Build history of the part. All positions in model axes, mm. Face numbers are marked on the shaded views. Coordinates: 2 decimals unless noted, no trailing zeros. Order: outer loops, then holes, each group sorted by start corner. A loop starts at its lowest first (then second) coordinate and runs counter-clockwise, first axis right, second up. Notation, with made-up numbers: (72.25, 44.5) - (93.25, 44.5) arc R25 ccw to (93.25, 74.5) - close; hole circle Ø8 at (-13.5, 46). An arc over 180 degrees is marked (long way). Return JSON: item names as keys, results as strings.
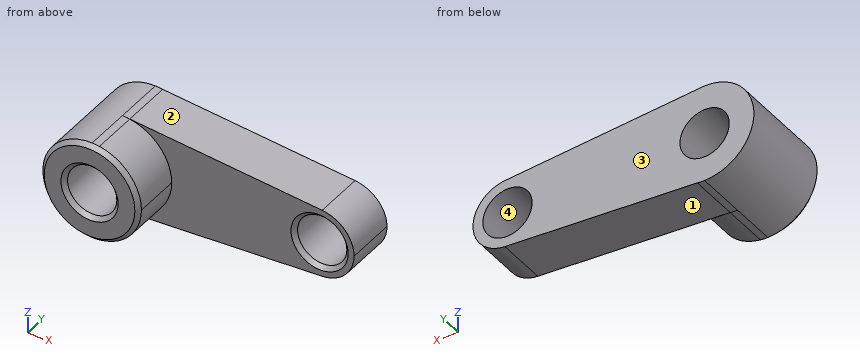
from build123d import *

# Parameters (mm, degrees)
F0_R        = 12.5
F1_DEPTH    = 25
F2_DEPTH    = 50
F3_T4_ANGLE = 203.6133668192
F3_T6_ANGLE = 179.9906971182


# Not quite as in the source:
# - a fillet or chamfer that OpenCascade refuses, or shapes differently, is made with other operations: its cross-section is extruded or revolved along the edge and cut away or added


with BuildPart() as f1:
    # F0 (on Front) → F1 (new body)
    with BuildSketch(Plane.XZ):
        with BuildLine():
            Line((3.7051688109, 24.7239099675), (0, 25))
            ThreePointArc((0, 25), (-25, 0), (0, -25))
            Line((0, -25), (3.7051688109, -24.7239099675))
            ThreePointArc((3.7051688109, -24.7239099675), (18.9424024383, -16.3151889313), (25, 0))
            ThreePointArc((25, 0), (18.9424024383, 16.3151889313), (3.7051688109, 24.7239099675))
        make_face()
        Circle(F0_R, mode=Mode.SUBTRACT)
        with BuildLine():
            ThreePointArc((3.7051688109, 24.7239099675), (1.8577204864, 24.9308819458), (0, 25))
            Line((0, 25), (3.7051688109, 24.7239099675))
        make_face()
        with BuildLine():
            Line((3.7051688109, -24.7239099675), (0, -25))
            ThreePointArc((0, -25), (1.8577204864, -24.9308819458), (3.7051688109, -24.7239099675))
        make_face()
        with BuildLine():
            Line((101.3004043405, 17.451617362), (3.7051688109, 24.7239099675))
            ThreePointArc((3.7051688109, 24.7239099675), (18.9424024383, 16.3151889313), (25, 0))
            ThreePointArc((25, 0), (18.9424024383, -16.3151889313), (3.7051688109, -24.7239099675))
            Line((3.7051688109, -24.7239099675), (101.3004043405, -17.451617362))
            ThreePointArc((101.3004043405, -17.451617362), (82.5, 0), (101.3004043405, 17.451617362))
        make_face()
        with BuildLine():
            ThreePointArc((117.5, 0), (112.8258932624, 11.9057323177), (101.3004043405, 17.451617362))
            ThreePointArc((101.3004043405, 17.451617362), (82.5, 0), (101.3004043405, -17.451617362))
            ThreePointArc((101.3004043405, -17.451617362), (112.8258932624, -11.9057323177), (117.5, 0))
        make_face()
        with Locations((100, 0)):
            Circle(F0_R, mode=Mode.SUBTRACT)
    extrude(amount=F1_DEPTH)

    # F0 (on Front) → F2 (join)
    with BuildSketch(Plane.XZ):
        with BuildLine():
            Line((3.7051688109, 24.7239099675), (0, 25))
            ThreePointArc((0, 25), (-25, 0), (0, -25))
            Line((0, -25), (3.7051688109, -24.7239099675))
            ThreePointArc((3.7051688109, -24.7239099675), (18.9424024383, -16.3151889313), (25, 0))
            ThreePointArc((25, 0), (18.9424024383, 16.3151889313), (3.7051688109, 24.7239099675))
        make_face()
        Circle(F0_R, mode=Mode.SUBTRACT)
    extrude(amount=F2_DEPTH)

    # F3: chamfer of 2 on 4 edges, made by hand

    # F3_s1 → F3_t2 (revolve, cut)
    with BuildSketch(Plane.XY):
        Polygon((14.5, -50), (12.5, -48), (12.5, -50), align=None)
    revolve(axis=Axis((0, -50, 0), (0, -1, 0)), mode=Mode.SUBTRACT)

    # F3_s3 → F3_t4 (revolve, cut)
    with BuildSketch(Plane(origin=(0, 0, 0), x_dir=(0, 1, 0), z_dir=(0.9788435281, 0, -0.2046102329))):
        Polygon((-48, 25), (-50, 23), (-50, 25), align=None)
    revolve(axis=Axis((0, -50, 0), (0, -1, 0)), revolution_arc=F3_T4_ANGLE, mode=Mode.SUBTRACT)

    # F3_s5 → F3_t6 (revolve, cut)
    with BuildSketch(Plane(origin=(0, 0, 0), x_dir=(0, 1, 0), z_dir=(-0.9999999967, 0, 8.1183e-05))):
        Polygon((-48, -25), (-50, -23), (-50, -25), align=None)
    revolve(axis=Axis((0, -50, 0), (0, 1, 0)), revolution_arc=F3_T6_ANGLE, mode=Mode.SUBTRACT)

    # F3_s7 → F3_t8 (revolve, cut)
    with BuildSketch(Plane.XY):
        Polygon((114.5, -25), (112.5, -23), (112.5, -25), align=None)
    revolve(axis=Axis((100, -25, 0), (0, -1, 0)), mode=Mode.SUBTRACT)


solid = f1.part
1. Drop flat-ended pins along their axis: pin 1 (4 mm diameter, centred on x = -10, z = -2, fed in from +Y); pin 2 (3 mm diameter, centred on x = 58.5, z = -16.5, fed in from -Y); pin 3 (4 mm diameter, centred on y = -30, z = -4, fed in from +X); pin 4 (2 mm diameter, centred on y = -45, z = 8.5, fed in from -X). Give the stop position or say it passes through.
Check values:
{"pin 1": "through", "pin 2": "y = -25", "pin 3": "x = 24.92", "pin 4": "x = -23.85"}
2. Cut at A-A on y = -34. Give the cut face in (x, z).
Check values:
{"outline": "(0, -25) - (3.71, -24.72) arc R25 ccw to (3.71, 24.72) - (0, 25) arc R25 ccw to start; hole circle Ø25 at (0, 0)"}
3. Mould opens along Z. For the marked faces 1, 2, 3 and 4 say: pulls with the +Z half, pulls with the -Z half, needs draft (parallel to the pull), parting line crosses it, or undercut.
Check values:
{"face 1": "pulls with the -Z half", "face 2": "pulls with the +Z half", "face 3": "needs draft", "face 4": "undercut"}
4. Cut at C-C on x = 100. Give the cut face in (y, z).
Check values:
{"outline": "(-25, -17.55) - (0, -17.55) - (0, -12.5) - (-23, -12.5) - (-25, -14.5) - close; (-25, 14.5) - (-23, 12.5) - (0, 12.5) - (0, 17.55) - (-25, 17.55) - close"}
5. Cut at D-D on z = -11. State how many separate pieces and enclosed holes the cut face has, plus the area to 3 significant figures.
Check values:
{"separate pieces": "3", "enclosed holes": "0", "area": "3,610 mm²"}
6. Cut at B-B on y = -17.5. Give the cut face in (x, z), plus the area to 3 significant figures.
Check values:
{"outline": "(3.71, -24.72) - (101.3, -17.45) arc R17.5 ccw to (101.3, 17.45) - (3.71, 24.72) arc R25 ccw (long way) to start; hole circle Ø25 at (0, 0); hole circle Ø25 at (100, 0)", "area": "4,740 mm²"}
7. Probe L1, parallel to X at y = -22, z = -9; L2, parallel to Y at x = 74.5, z = 14; L3, parallel to X at y = -41.5, z = -1. List the from-to ranges inside material, lowest first.
Check values:
{"L1": "-23.32 to -8.67, 8.67 to 91.33, 108.67 to 115.01", "L2": "-25 to 0", "L3": "-24.98 to -12.46, 12.46 to 24.98"}
